Design review of the part shown in the three views and the two pictorial views. Dimensions are in mm from the part's minimum x, y and z. A direction names the side the tool comes from. Coordinates: 2 decimals unless noted, no trailing zeros. Order: outer loops, then holes, each group sorted by start corner. A loop starts at its lowest first (then second) coordinate and runs counter-clockwise, first axis right, second up. Notation, with made-up numbers: (41.25, 54.25) -> (61.25, 54.25) arc R5 ccw to (61.25, 59.25) -> close; hole circle Ø9 at (15, -31). An arc over 180 degrees is marked (long way). Answer as CSV lines item,"result". Start each with the question number.
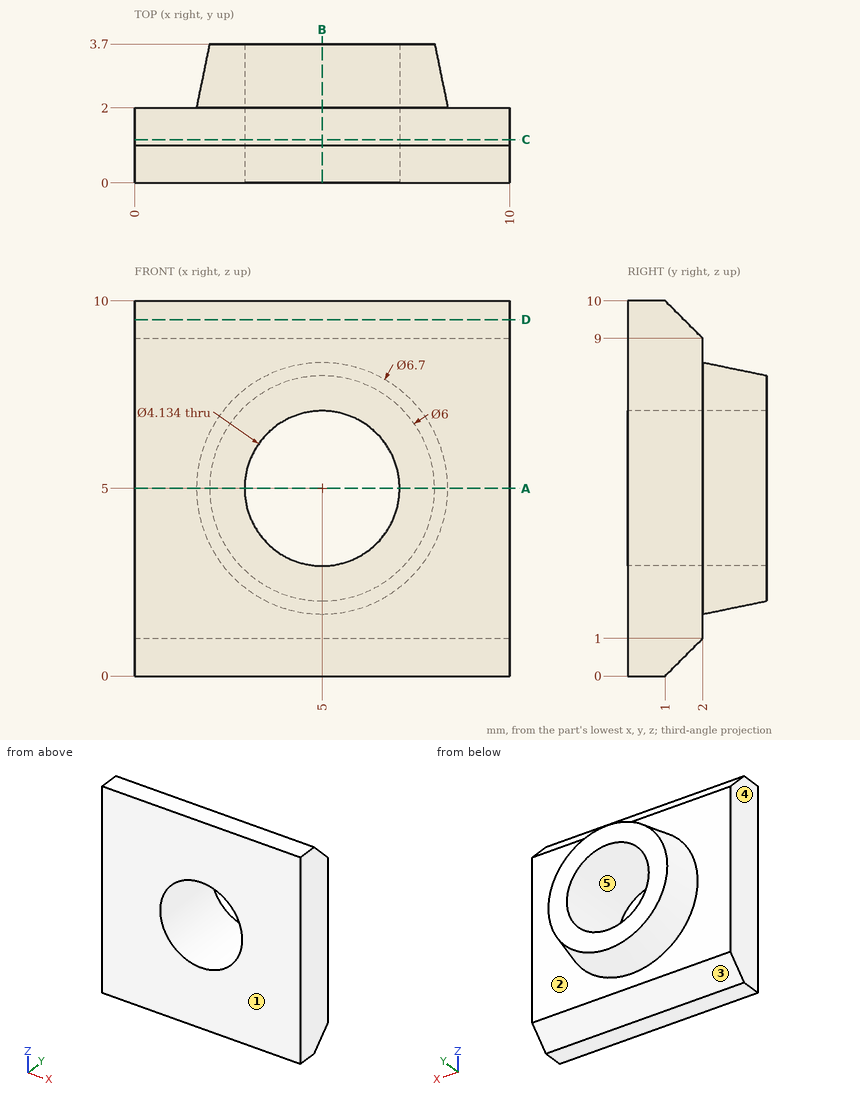
1) Consider section A-A (z = 5). Give the boundary of the cut face in (x, y).
2) Consider section D-D (z = 9.5). Give the boundary of the cut face in (x, y).
3) Consider section B-B (x = 5). Give the boundary of the cut face in (y, z), plus the area to 3 significant figures.
4) Tool access review of the marked faces 1 and 2: name each direction out of +Z, -Z, +X, -X, +Y, -Y from which nothing blocks a thin tool from reaching the whole face with its end or side.
5) Wall thickness on L1, parallel to Y at x = 3.75, z = 8.5; L2, parallel to Z at x = 5, y = 2.4; L3, parallel to X at y = 2.1, z = 5.5: over which ranges is each line inside the solid? List them lowest first. Write a range as [from, to].
6) Consider section C-C (y = 1.15). Give the boundary of the cut face in (x, z), plus the area to 3 significant figures.
7) Mouldability with a two-part tool opening along Z and no side actions: class the marked faces 3, 4 and 5 as released by +Z, released by -Z, zero draft, split by the parting line, or undercut.
Result:
1,outline,"(0, 0) -> (2.93, 0) -> (2.93, 3.7) -> (2, 3.7) -> (1.65, 2) -> (0, 2) -> close; (7.07, 0) -> (10, 0) -> (10, 2) -> (8.35, 2) -> (8, 3.7) -> (7.07, 3.7) -> close"
2,outline,"(0, 0) -> (10, 0) -> (10, 1.5) -> (0, 1.5) -> close"
3,outline,"(0, 0) -> (1, 0) -> (2, 1) -> (2, 1.65) -> (3.7, 2) -> (3.7, 2.93) -> (0, 2.93) -> close; (0, 7.07) -> (3.7, 7.07) -> (3.7, 8) -> (2, 8.35) -> (2, 9) -> (1, 10) -> (0, 10) -> close"
3,area,"14.5 mm2"
4,face 1,"+Z, -Z, +X, -X, -Y"
4,face 2,"+Y"
5,L1,"[0, 2]"
5,L2,"[1.73, 2.93], [7.07, 8.27]"
5,L3,"[1.71, 2.99], [7.01, 8.29]"
6,outline,"(0, 0.15) -> (10, 0.15) -> (10, 9.85) -> (0, 9.85) -> close; hole circle Ø4.13 at (5, 5)"
6,area,"83.6 mm2"
7,face 3,"released by -Z"
7,face 4,"zero draft"
7,face 5,"undercut"
